from build123d import *

# Parameters (mm, degrees)
F0_W     = 88.9
F0_H     = 38.1
F1_DEPTH = 635
F2_W     = 88.9
F2_H     = 38.1
F3_DEPTH = 19.05


# Not quite as in the source:
# - a length typed as a fraction of an inch, garbled in the dataset ("3 / 203.2 mm" for 3/8 in), is restored


with BuildPart() as f1:
    # F0 (on Front) → F1 (new body, symmetric)
    with BuildSketch(Plane.XZ):
        Rectangle(F0_W, F0_H)
    extrude(amount=F1_DEPTH, both=True)

    # F2 (on face) → F3 (cut)
    with BuildSketch(Plane.XY.offset(19.05)):
        with Locations((0, 527.05)):
            Rectangle(F2_W, F2_H)
        with Locations((0, -527.05)):
            Rectangle(F2_W, F2_H)
    extrude(amount=-F3_DEPTH, mode=Mode.SUBTRACT)


solid = f1.part
The model under review builds one solid part; all positions refer to its coordinate system, in mm. A direction names the side the tool comes from. Coordinates: 2 decimals unless noted, no trailing zeros. Write each loop counter-clockwise with the first axis right and the second up, starting at its lowest first coordinate (ties: lowest second). Pieces come first, ordered by that corner, then holes. Notation, with made-up numbers: (-10.5, 2.5) - (42.5, 2.5) arc R27 ccw to (42.5, 39.5) - close; hole circle Ø5 at (-33.5, -32.5). An arc over 180 degrees is marked (long way). Answer as a JSON object with one key per item and string values. Group by question number.
1. Mouldability with a two-part tool opening along Y and no side actions: class faces 1 (the face through (-1, -591, 19.05)), 2 (the face through (-1, 527, 0)), 3 (the face through (-1, 635, 0)) as pulls with the +Y half, pulls with the -Y half, needs draft (parallel to the pull), parting line crosses it, or undercut.
2. Add section A-A (x = 15.5). Give the boundary of the cut face in (y, z).
3. To check wall thickness, follow probe 1 along Y at (x, z) = (-13, 16.5); probe 2 along Z at (x, y) = (17, -543.5). State the ranges of each line that lie inside material, in increasing order.
4. Machinability: for faces 4 (the face through (-1, -527, 0)), 5 (the face through (-1, -7, 19.05)), which of the approach directions +Z, -Z, +X, -X, +Y, -Y give a long, thin tool a straight path to every point of the face, cutting with its end or side? Answer none if there is none.
Findings:
{
 "1": {"face 1": "needs draft", "face 2": "undercut", "face 3": "pulls with the +Y half"},
 "2": {"outline": "(-635, -19.05) - (635, -19.05) - (635, 19.05) - (546.1, 19.05) - (546.1, 0) - (508, 0) - (508, 19.05) - (-508, 19.05) - (-508, 0) - (-546.1, 0) - (-546.1, 19.05) - (-635, 19.05) - close"},
 "3": {"probe 1": "-635 to -546.1, -508 to 508, 546.1 to 635", "probe 2": "-19.05 to 0"},
 "4": {"face 4": "+Z, +X, -X", "face 5": "+Z, +X, -X, +Y, -Y"}
}
